For this review, take the finished solid that the model builds, in its own axes (mm). Face numbers are marked on the shaded views. A direction names the side the tool comes from. Round coordinates to 2 decimals unless told otherwise and drop trailing zeros. Write each loop counter-clockwise with the first axis right and the second up, starting at its lowest first coordinate (ties: lowest second). Pieces come first, ordered by that corner, then holes. Notation, with made-up numbers: (-31, 75) -> (1, 75) arc R24 ccw to (1, 88) -> close; hole circle Ø4 at (-10.75, -3). An arc over 180 degrees is marked (long way). Answer in a Markdown table with one row per item. Add a question column.
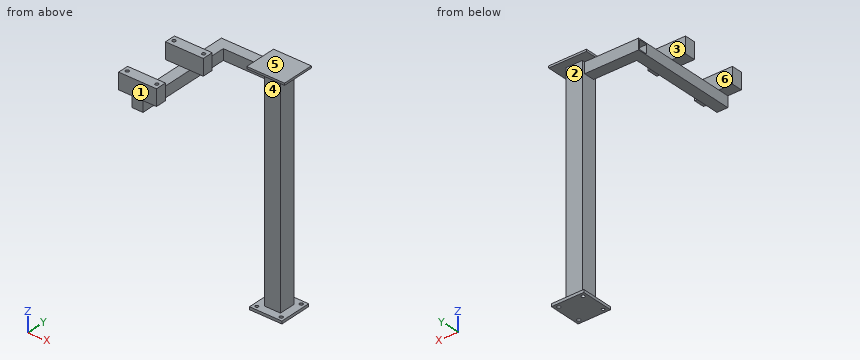
```python
from build123d import *

# Parameters (mm, degrees)
F0_W      = 152.4
F0_H      = 152.4
F1_DEPTH  = 12.7
F2_W      = 76.2
F2_H      = 76.2
F2_W_2    = 63.5
F2_H_2    = 63.5
F3_DEPTH  = 1016
F4_W      = 41.275
F4_H      = 41.275
F5_DEPTH  = 254
F6_W      = 50.8
F6_H      = 50.8
F7_DEPTH  = 457.2
F8_W      = 177.8
F8_H      = 50.8
F9_DEPTH  = 76.2
F11_DEPTH = 9.525
F13_DEPTH = 19.05
F15_DEPTH = 19.05
F16_R     = 7.9375
F17_DEPTH = 25.4


with BuildPart() as f1:
    # F0 (on Top) → F1 (new body)
    with BuildSketch(Plane.XY):
        with Locations((76.2, 76.2)):
            Rectangle(F0_W, F0_H)
    extrude(amount=F1_DEPTH)

    # F2 (on face) → F3 (join)
    with BuildSketch(Plane.XY.offset(12.7)):
        with Locations((76.2, 76.2)):
            Rectangle(F2_W, F2_H)
        with Locations((76.2, 76.2)):
            Rectangle(F2_W_2, F2_H_2, mode=Mode.SUBTRACT)
    extrude(amount=F3_DEPTH)

    # F4 (on face) → F5 (join)
    with BuildSketch(Plane(origin=(38.1, 0, 0), x_dir=(0, -1, 0), z_dir=(-1, 0, 0))):
        Polygon((-50.8, 1028.7), (-101.6, 1028.7), (-101.6, 1023.9375), (-101.6, 977.9), (-50.8, 977.9), align=None)
        with Locations((-76.2, 1003.3)):
            Rectangle(F4_W, F4_H, mode=Mode.SUBTRACT)
    extrude(amount=F5_DEPTH)

    # F6 (on face) → F7 (join)
    with BuildSketch(Plane.XZ.offset(-50.8)):
        with Locations((-190.5, 1003.3)):
            Rectangle(F6_W, F6_H)
    extrude(amount=F7_DEPTH)

    # F8 (on face) → F9 (join)
    with BuildSketch(Plane.XY.offset(1028.7)):
        with Locations((-190.5, -381)):
            Rectangle(F8_W, F8_H)
        Polygon((-101.6, -88.9), (-165.1, -88.9), (-279.4, -88.9), (-279.4, -139.7), (-101.6, -139.7), align=None)
    extrude(amount=F9_DEPTH)

    # F10 (on face) → F11 (join)
    with BuildSketch(Plane.XY.offset(1028.7)):
        Polygon((165.1, 152.4), (114.3, 152.4), (-12.7, 152.4), (-12.7, 0), (165.1, 0), align=None)
    extrude(amount=F11_DEPTH)

    # F12 (on face) → F13 (cut)
    with BuildSketch(Plane.XY.offset(1104.9)):
        with BuildLine():
            Line((-268.2875, -114.3), (-260.35, -114.3))
            Line((-260.35, -114.3), (-252.4125, -114.3))
            ThreePointArc((-252.4125, -114.3), (-260.35, -106.3625), (-268.2875, -114.3))
        make_face()
        with BuildLine():
            Line((-252.4125, -114.3), (-260.35, -114.3))
            Line((-260.35, -114.3), (-268.2875, -114.3))
            ThreePointArc((-268.2875, -114.3), (-260.35, -122.2375), (-252.4125, -114.3))
        make_face()
        with BuildLine():
            ThreePointArc((-112.7125, -114.3), (-120.65, -106.3625), (-128.5875, -114.3))
            Line((-128.5875, -114.3), (-120.65, -114.3))
            Line((-120.65, -114.3), (-112.7125, -114.3))
        make_face()
        with BuildLine():
            Line((-120.65, -114.3), (-128.5875, -114.3))
            ThreePointArc((-128.5875, -114.3), (-120.65, -122.2375), (-112.7125, -114.3))
            Line((-112.7125, -114.3), (-120.65, -114.3))
        make_face()
    extrude(amount=-F13_DEPTH, mode=Mode.SUBTRACT)

    # F14 (on face) → F15 (cut)
    with BuildSketch(Plane.XY.offset(1104.9)):
        with BuildLine():
            Line((-268.2875, -381), (-260.35, -381))
            Line((-260.35, -381), (-252.4125, -381))
            ThreePointArc((-252.4125, -381), (-260.35, -373.0625), (-268.2875, -381))
        make_face()
        with BuildLine():
            Line((-252.4125, -381), (-260.35, -381))
            Line((-260.35, -381), (-268.2875, -381))
            ThreePointArc((-268.2875, -381), (-260.35, -388.9375), (-252.4125, -381))
        make_face()
        with BuildLine():
            ThreePointArc((-112.7125, -381), (-120.65, -373.0625), (-128.5875, -381))
            Line((-128.5875, -381), (-120.65, -381))
            Line((-120.65, -381), (-112.7125, -381))
        make_face()
        with BuildLine():
            Line((-120.65, -381), (-128.5875, -381))
            ThreePointArc((-128.5875, -381), (-120.65, -388.9375), (-112.7125, -381))
            Line((-112.7125, -381), (-120.65, -381))
        make_face()
    extrude(amount=-F15_DEPTH, mode=Mode.SUBTRACT)

    # F16 (on face) → F17 (cut)
    with BuildSketch(Plane.XY.offset(12.7)):
        with BuildLine():
            ThreePointArc((19.05, 11.90625), (24.101394, 13.998606), (26.19375, 19.05))
            ThreePointArc((26.19375, 19.05), (13.998606, 24.101394), (19.05, 11.90625))
        make_face()
        with BuildLine():
            ThreePointArc((133.35, 141.2875), (127.73734, 127.73734), (141.2875, 133.35))
            ThreePointArc((141.2875, 133.35), (138.96266, 138.96266), (133.35, 141.2875))
        make_face()
        with Locations((133.35, 19.05)):
            Circle(F16_R)
        with BuildLine():
            ThreePointArc((19.05, 141.2875), (13.43734, 127.73734), (26.9875, 133.35))
            ThreePointArc((26.9875, 133.35), (24.66266, 138.96266), (19.05, 141.2875))
        make_face()
    extrude(amount=-F17_DEPTH, mode=Mode.SUBTRACT)


solid = f1.part
```
1. Clearance check with flat-ended pins moving along their axes: pin 1 Ø10.5 at (x, z) = (51.5, 1034.5) entering from -Y; pin 2 Ø18.5 at (x, y) = (-120.65, -114.3) entering from -Z; pin 3 Ø8 at (x, y) = (-180.5, -161) entering from +Z; pin 4 Ø5 at (x, z) = (32, 973) entering from +Y. State where each tip first meets the part, or that it passes through.
2. For L1, parallel to Y at x = 133.35, z = 9.25; L2, parallel to X at y = -114.3, z = 1096.5; L3, parallel to Z at x = 12, y = 91 (1 decimal), list the stretches that pass through material, from the lowest coordinate up. Write a range as [from, to].
3. We need section C-C (y = -318). Write out the cut boundary in (x, z), plus the area to 3 significant figures.
4. The part is to be moulded in two halves that separate along Z. For the marked faces 4, 5 and 6, say which applies: pulls with the +Z half, pulls with the -Z half, needs draft (parallel to the pull), parting line crosses it, or undercut.
5. We need section A-A (z = 827). Write out the cut boundary in (x, y).
6. We need section B-B (x = -200). Write out the cut boundary in (y, z), plus the area to 3 significant figures.
7. Tool access review of the marked faces 1, 2 and 3: name each direction out of +Z, -Z, +X, -X, +Y, -Y from which nothing blocks a thin tool from reaching the whole face with its end or side.
Response:
| question | item | result |
|---|---|---|
| 1 | pin 1 | y = 0 |
| 1 | pin 2 | z = 1028.7 |
| 1 | pin 3 | z = 1028.7 |
| 1 | pin 4 | through |
| 2 | L1 | [0, 11.11], [26.99, 125.41], [141.29, 152.4] |
| 2 | L2 | [-279.4, -268.29], [-252.41, -128.59], [-112.71, -101.6] |
| 2 | L3 | [0, 12.7], [977.9, 982.7], [1023.9, 1038.2] |
| 3 | outline | (-215.9, 977.9) -> (-165.1, 977.9) -> (-165.1, 1028.7) -> (-215.9, 1028.7) -> close |
| 3 | area | 2,580 mm2 |
| 4 | face 4 | undercut |
| 4 | face 5 | pulls with the +Z half |
| 4 | face 6 | needs draft |
| 5 | outline | (38.1, 38.1) -> (114.3, 38.1) -> (114.3, 114.3) -> (38.1, 114.3) -> close; hole (44.45, 44.45) -> (107.95, 44.45) -> (107.95, 107.95) -> (44.45, 107.95) -> close |
| 6 | outline | (-406.4, 977.9) -> (101.6, 977.9) -> (101.6, 1028.7) -> (-88.9, 1028.7) -> (-88.9, 1104.9) -> (-139.7, 1104.9) -> (-139.7, 1028.7) -> (-355.6, 1028.7) -> (-355.6, 1104.9) -> (-406.4, 1104.9) -> close; hole (55.56, 982.66) -> (96.84, 982.66) -> (96.84, 1023.94) -> (55.56, 1023.94) -> close |
| 6 | area | 31,800 mm2 |
| 7 | face 1 | +Z, -Z, +X, -X, -Y |
| 7 | face 2 | +X, -X, +Y |
| 7 | face 3 | +Z, +X, -X, +Y |
